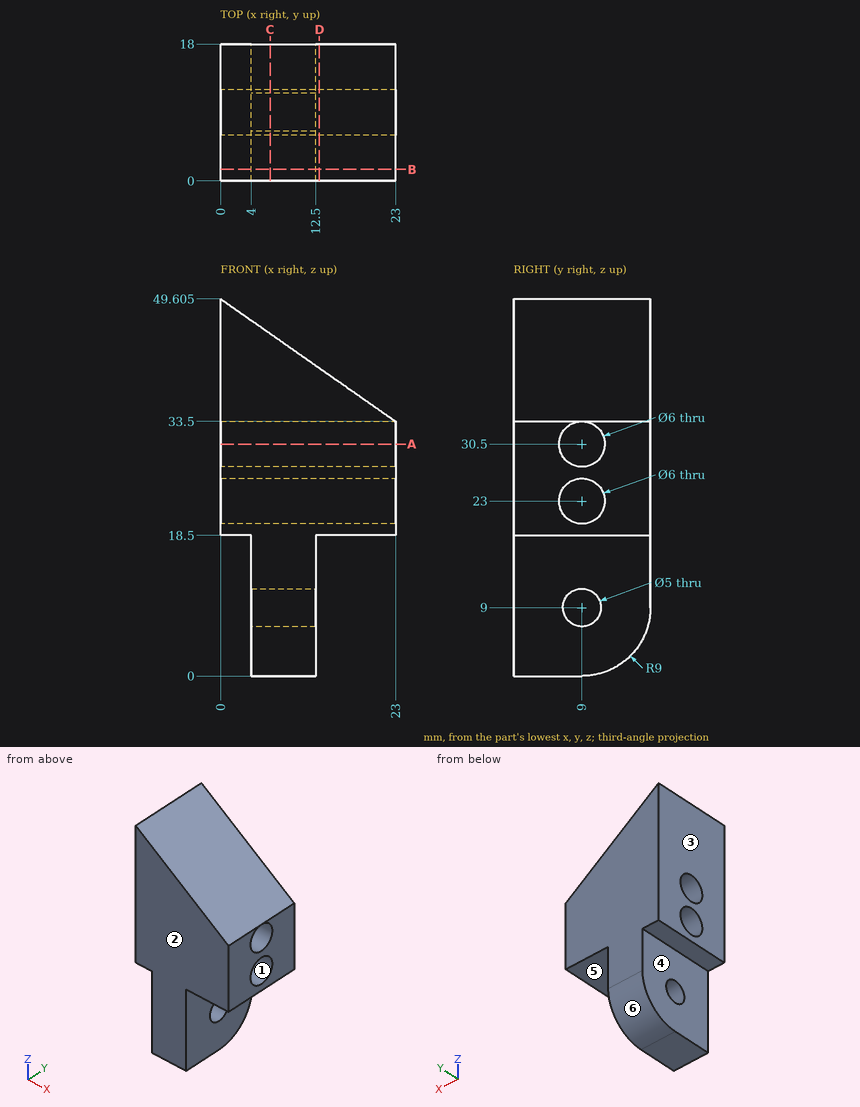
Study the drawing (mm; zero at the part's minimum x, y, z) and answer. A direction names the side the tool comes from. Give positions to 0.01 mm unless a question says otherwise; leave off trailing zeros. Order: outer loops, then holes, each group sorted by start corner. A loop starts at its lowest first (then second) coordinate and runs counter-clockwise, first axis right, second up.
1. For the marked faces 4, 5 and 6, determine the directions among +Z, -Z, +X, -X, +Y, -Y from which every point of the face is accessible in a straight line to the end or side of a thin tool.
Result sheet:
face 4: -Z, -X, +Y, -Y
face 5: -Z, +X, +Y, -Y
face 6: -Z, +X, -X, +Y
2. Section B-B, the plane y = 1.5 is taken. Determine the outline of the cut face in (x, z) (1 decimal).
Result sheet:
outline: (0, 18.5) - (4, 18.5) - (4, 0) - (12.5, 0) - (12.5, 18.5) - (23, 18.5) - (23, 33.5) - (0, 49.6) - close
3. Section C-C, the plane x = 6.5 is taken. Determine the outline of the cut face in (y, z), and give its area (3 significant figures).
Result sheet:
outline: (0, 0) - (9, 0) arc R9 ccw to (18, 9) - (18, 45.05) - (0, 45.05) - close; hole circle Ø6 at (9, 23); hole circle Ø6 at (9, 30.5); hole circle Ø5 at (9, 9)
area: 717 mm2
4. The mould has two halves that part along Y. Classify the marked faces 1, 2 and 3: released by +Y, released by -Y, zero draft, split by the parting line, or undercut.
Result sheet:
face 1: undercut
face 2: released by -Y
face 3: zero draft
5. Straight lines are drawn through the part: L1, parallel to Y at x = 7.25, z = 30.5; L2, parallel to Z at x = 18, y = 11 (1 decimal); L3, parallel to Z at x = 14.25, y = 9.25. For each, find the intervals that lie inside material, in ascending order.
Result sheet:
L1: y = 0 to 6, 12 to 18
L2: z = 18.5 to 20.8, 25.2 to 28.3, 32.7 to 37
L3: z = 18.5 to 20.01, 25.99 to 27.51, 33.49 to 39.63
6. Section A-A, the plane z = 30.5 is taken. Determine the outline of the cut face in (x, y), and give its area (3 significant figures).
Result sheet:
outline: (0, 0) - (23, 0) - (23, 6) - (0, 6) - close; (0, 12) - (23, 12) - (23, 18) - (0, 18) - close
area: 276 mm2
7. Section D-D, the plane x = 13 is taken. Determine the outline of the cut face in (y, z).
Result sheet:
outline: (0, 18.5) - (18, 18.5) - (18, 40.5) - (0, 40.5) - close; hole circle Ø6 at (9, 23); hole circle Ø6 at (9, 30.5)
8. Each of these flat-tipped pins is pushed along its axis until it touches: P1, Ø10, axis at y = 13, z = 13, coming from the -X side; P2, Ø5.5, axis at y = 9, z = 30.5, coming from the -X side; P3, Ø3, axis at y = 2.5, z = 12, coming from the +X side; P4, Ø8, axis at y = 2, z = 42.5, coming from the +X side. Where does it stop, or does it pass through?
Result sheet:
P1: stops at x = 4
P2: passes through
P3: stops at x = 12.5
P4: stops at x = 15.86
